Could you check a few things on this drawing? It's one solid part, dimensions in mm from its lowest x, y, z. A direction names the side the tool comes from. Coordinates: 2 decimals unless noted, no trailing zeros. Write each loop counter-clockwise with the first axis right and the second up, starting at its lowest first coordinate (ties: lowest second). Pieces come first, ordered by that corner, then holes. Notation, with made-up numbers: (-15.75, 60.25) - (-8.75, 60.25) arc R16 ccw to (-8.75, 89.25) - close; hole circle Ø6 at (-9, -3). An arc over 180 degrees is marked (long way). Answer as a JSON object with one key per item and string values. Group by question number.
1) Please list where these lines run through material, in increasing order: line 1 along Y through (x, z) = (7.5, 1.75); line 2 along X through (y, z) = (4.25, 11.75); line 3 along X through (y, z) = (2.25, 2).
2) If we section it at D-D (y = 4.5): Write out the boundary of the cut face in (x, z) (3 decimals), plus the area to 3 significant figures.
3) If we section it at C-C (y = 18): Write out the boundary of the cut face in (x, z) (3 decimals).
4) Will these pins go through, and if not, where does the flat tip stop? pin 1 Ø2 at (y, z) = (10.5, 10.5) entering from +X; pin 2 Ø1 at (x, y) = (13.5, 13.5) entering from +Z; pin 3 Ø1 at (x, y) = (20.5, 12) entering from -Z.
5) We'd pull the mould along Y, two halves only. Please class the marked faces 3, 4, 5 and 6: released by +Y, released by -Y, zero draft, split by the parting line, or undercut.
6) On a 3-axis mill with a long thin cutter (end or side, diameter ignored), from which of +Z, -Z, +X, -X, +Y, -Y can I reach the whole of each face in a straight line? I mean the marked faces 1 and 2. Say none if no direction works.
7) If we section it at A-A (z = 21): Write out the boundary of the cut face in (x, y).
8) If we section it at B-B (x = 14.5): Write out the boundary of the cut face in (y, z).
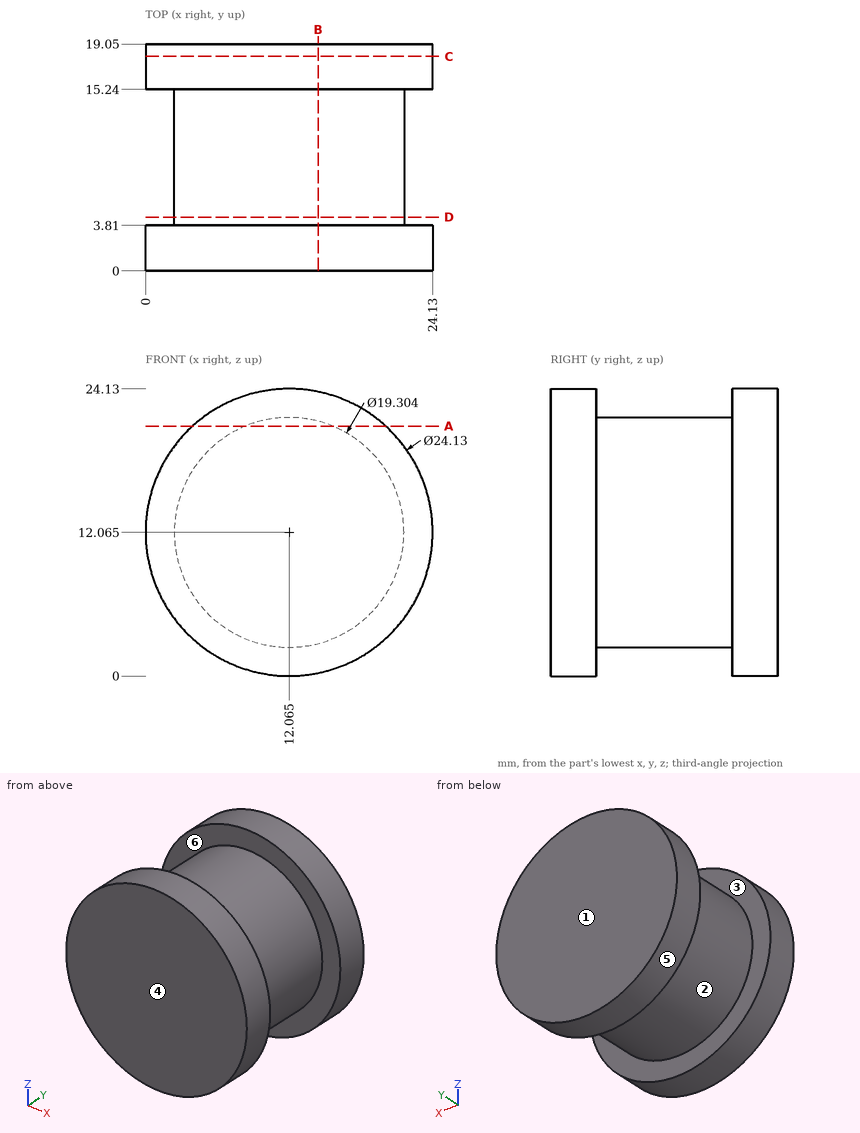
Here are the results:
{
 "1": {"line 1": "y = 0 to 3.81, 15.24 to 19.05", "line 2": "x = 2.42 to 21.71", "line 3": "x = 5.41 to 18.72"},
 "2": {"outline": "circle Ø19.304 at (12.065, 12.065)", "area": "293 mm²"},
 "3": {"outline": "circle Ø24.13 at (12.065, 12.065)"},
 "4": {"pin 1": "stops at x = 21.7", "pin 2": "stops at z = 21.67", "pin 3": "stops at z = 6.57"},
 "5": {"face 3": "undercut", "face 4": "released by -Y", "face 5": "zero draft", "face 6": "undercut"},
 "6": {"face 1": "+Z, -Z, +X, -X, +Y", "face 2": "none"},
 "7": {"outline": "(3.96, 0) - (20.17, 0) - (20.17, 3.81) - (15.72, 3.81) - (15.72, 15.24) - (20.17, 15.24) - (20.17, 19.05) - (3.96, 19.05) - (3.96, 15.24) - (8.41, 15.24) - (8.41, 3.81) - (3.96, 3.81) - close"},
 "8": {"outline": "(0, 0.25) - (3.81, 0.25) - (3.81, 2.73) - (15.24, 2.73) - (15.24, 0.25) - (19.05, 0.25) - (19.05, 23.88) - (15.24, 23.88) - (15.24, 21.4) - (3.81, 21.4) - (3.81, 23.88) - (0, 23.88) - close"}
}
